Check sheet for the modelled part. Datum: model origin and axes. Units: mm. Face numbers are marked on the shaded views. A direction names the side the tool comes from. Give positions to 0.01 mm unless a question says otherwise; leave off trailing zeros. Order: outer loops, then holes, each group sorted by start corner. A loop starts at its lowest first (then second) coordinate and runs counter-clockwise, first axis right, second up. Notation, with made-up numbers: (65, 41.25) -> (84, 41.25) arc R29 cw to (84, 74.25) -> close; hole circle Ø11 at (-9.75, 55). An arc over 180 degrees is marked (long way). Answer in a Markdown table with one row per item. Add a question column.
(1) Go/stop test with flat-tipped pins: pin 1 (1 mm diameter, centred on x = 1.5, z = -20.5, fed in from -Y); pin 2 (4 mm diameter, centred on x = -0.5, z = -16.5, fed in from -Y); pin 3 (8 mm diameter, centred on y = -0.5, z = -91, fed in from +X). Record where each tip stops, or that it passes through.
(2) Cross-section at C-C (z = -40). Record the cut outline in (x, y).
(3) Thickness scan on L1, parallel to Y at x = 0.5, z = -109; L2, parallel to Z at x = 6.5, y = -2.5; L3, parallel to Z at x = 5, y = -11. Record the ranges inside material, lowest first. Write a range as [from, to].
(4) Cross-section at D-D (y = -15). Record the cut outline in (x, z).
(5) Cross-section at A-A (x = 0). Record the cut outline in (y, z).
(6) Cross-section at B-B (y = 0). Record the cut outline in (x, z), then the cut area to 3 significant figures.
(7) Set-up check for the marked faces 1 and 2: record each of +Z, -Z, +X, -X, +Y, -Y from which the full face is reachable in a straight line by a thin tool's end or side.
```python
from build123d import *

# Parameters (mm, degrees)
F0_R     = 3
F3_DEPTH = 130
F4_DEPTH = 130
F5_START = 130
F2_R     = 10
F5_DEPTH = 20


with BuildPart() as f3:
    # F0 (on Top) → F3 (new body)
    with BuildSketch(Plane.XY):
        Circle(F0_R)
    extrude(amount=-F3_DEPTH)

    # F1 (on Top) → F4 (join)
    with BuildSketch(Plane.XY):
        Polygon((12.5, -12.5), (12.5, 12.5), (-12.5, 12.5), (-12.5, -12.5), (-12.5, -22.5), (12.5, -22.5), align=None)
    extrude(amount=F4_DEPTH)

    # F2 (on Top) → F5 (join)
    with BuildSketch(Plane.XY.offset(F5_START)):
        Circle(F2_R)
    extrude(amount=F5_DEPTH)


solid = f3.part
```
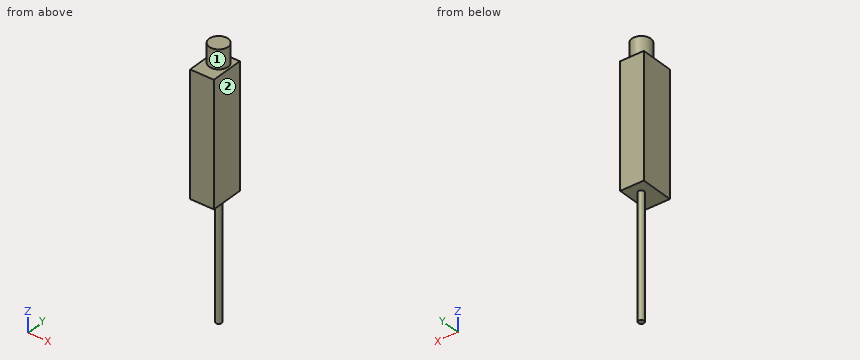
Answer below:
| question | item | result |
|---|---|---|
| 1 | pin 1 | stops at y = -2.83 |
| 1 | pin 2 | stops at y = -3 |
| 1 | pin 3 | stops at x = 3 |
| 2 | outline | circle Ø6 at (0, 0) |
| 3 | L1 | y = [-2.96, 2.96] |
| 3 | L2 | z = [0, 150] |
| 3 | L3 | z = [0, 130] |
| 4 | outline | (-12.5, 0) -> (12.5, 0) -> (12.5, 130) -> (-12.5, 130) -> close |
| 5 | outline | (-22.5, 0) -> (-3, 0) -> (-3, -130) -> (3, -130) -> (3, 0) -> (12.5, 0) -> (12.5, 130) -> (10, 130) -> (10, 150) -> (-10, 150) -> (-10, 130) -> (-22.5, 130) -> close |
| 6 | outline | (-12.5, 0) -> (-3, 0) -> (-3, -130) -> (3, -130) -> (3, 0) -> (12.5, 0) -> (12.5, 130) -> (10, 130) -> (10, 150) -> (-10, 150) -> (-10, 130) -> (-12.5, 130) -> close |
| 6 | area | 4,430 mm² |
| 7 | face 1 | +Z |
| 7 | face 2 | +Z, -Z, +X, +Y, -Y |
